```python
from build123d import *


with BuildPart() as part:
    # Croquis1 → Revolución1 (revolve)
    with BuildSketch(Plane(origin=(0, 0, 0), x_dir=(1, 0, 0), z_dir=(0, 1, 0))):
        Polygon((1.5, 1.013513514), (8.5, 1.013513514), (8.5, 22.8), (11, 22.8), (11, 22.6), (15.5, 22.6), (15.5, 0), (11, 0), (11, -0.2), (1.5, -0.2), align=None)
    revolve(axis=Axis((0, 0, 0), (0, 0, -1)))


solid = part.part
```
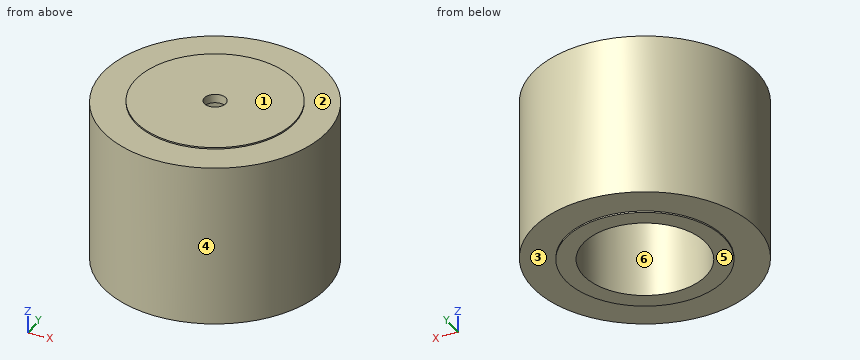
The listing builds one solid part. Answer for the finished solid, in the listing's coordinates (mm). Face numbers are marked on the shaded views. A direction names the side the tool comes from. Round coordinates to 2 decimals unless told otherwise and drop trailing zeros. Order: outer loops, then holes, each group sorted by start corner. A loop starts at its lowest first (then second) coordinate and runs counter-clockwise, first axis right, second up. Notation, with made-up numbers: (22, -22.75) - (53, -22.75) arc R20 ccw to (53, 8.25) - close; hole circle Ø1 at (87.25, -20). An arc over 180 degrees is marked (long way). Put each result on its own line as item: value. Start each with the question number.
(1) Find section A-A (y = 0). Give the vertices of the cut face in (x, z), plus the area to 3 significant figures.
(2) Find section D-D (x = 5). Give the vertices of the cut face in (y, z).
(3) Given P1, Ø6, axis at y = -3.5, z = -12, coming from the +X side; P2, Ø18.5, axis at x = -3.5, y = 0, coming from the -Z side; P3, Ø1.5, axis at x = 12, z = -14, coming from the +Y side; P4, Ø5, axis at x = -11, y = -9.5, coming from the +Z side, each flat-ended and moving along its own axis, determine where each tip first touches the part or whether it passes through.
(4) Determine the mould class of the marked faces 4, 5 and 6 for opening direction X: released by +X, released by -X, zero draft, split by the parting line, or undercut.
(5) For the marked faces 1, 2 and 3, determine the directions among +Z, -Z, +X, -X, +Y, -Y from which every point of the face is accessible in a straight line to the end or side of a thin tool.
(6) Find section C-C (y = -9). Give the vertices of the cut face in (x, z), plus the area to 3 significant figures.
(7) Straight lines are drawn through the part: probe 1 along Y at (x, z) = (0, -14); probe 2 along Y at (x, z) = (0, -0.65). For each, find the intervals that lie inside material, in ascending order. Write a range as from..to.
Reply:
1. outline: (-15.5, -22.6) - (-11, -22.6) - (-11, -22.8) - (-8.5, -22.8) - (-8.5, -1.01) - (-1.5, -1.01) - (-1.5, 0.2) - (-11, 0.2) - (-11, 0) - (-15.5, 0) - close; (1.5, -1.01) - (8.5, -1.01) - (8.5, -22.8) - (11, -22.8) - (11, -22.6) - (15.5, -22.6) - (15.5, 0) - (11, 0) - (11, 0.2) - (1.5, 0.2) - close
1. area: 335 mm^2
2. outline: (-14.67, -22.6) - (-9.8, -22.6) - (-9.8, -22.8) - (-6.87, -22.8) - (-6.87, -1.01) - (6.87, -1.01) - (6.87, -22.8) - (9.8, -22.8) - (9.8, -22.6) - (14.67, -22.6) - (14.67, 0) - (9.8, 0) - (9.8, 0.2) - (-9.8, 0.2) - (-9.8, 0) - (-14.67, 0) - close
3. P1: x = 15.49
3. P2: z = -22.8
3. P3: y = 10.66
3. P4: z = 0
4. face 4: split by the parting line
4. face 5: zero draft
4. face 6: undercut
5. face 1: +Z, +X, -X, +Y, -Y
5. face 2: +Z
5. face 3: -Z
6. outline: (-12.62, -22.6) - (-6.32, -22.6) - (-6.32, -22.8) - (6.32, -22.8) - (6.32, -22.6) - (12.62, -22.6) - (12.62, 0) - (6.32, 0) - (6.32, 0.2) - (-6.32, 0.2) - (-6.32, 0) - (-12.62, 0) - close
6. area: 575 mm^2
7. probe 1: -15.5..-8.5, 8.5..15.5
7. probe 2: -15.5..-1.5, 1.5..15.5
